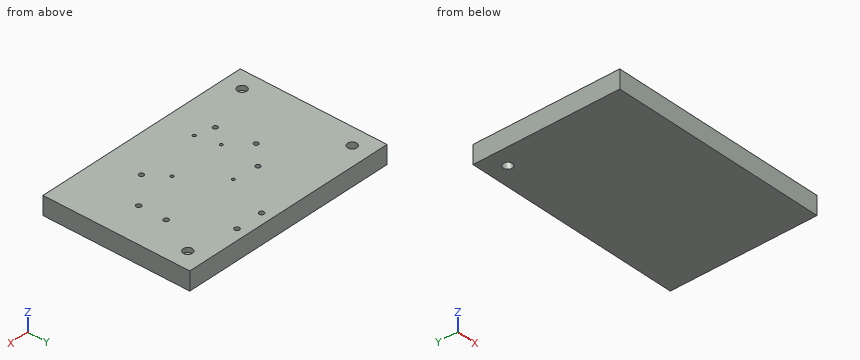
```python
from build123d import *

# Parameters (mm, degrees)
F0_W      = 304.8
F0_H      = 203.2
F1_DEPTH  = 25.4
F2_R      = 6.35
F3_DEPTH  = 6.35
F4_R      = 3.175
F5_DEPTH  = 19.05
F6_R      = 2.0701
F7_DEPTH  = 13.0302
F8_R      = 3.429
F9_DEPTH  = 12.7
F10_R     = 3.175
F11_DEPTH = 6.35
F12_R     = 3.429
F13_DEPTH = 12.7
F14_R     = 2.159
F15_DEPTH = 12.7
F16_R     = 6.35
F17_DEPTH = 25.4


with BuildPart() as f1:
    # F0 (on Top) → F1 (new body)
    with BuildSketch(Plane.XY):
        Rectangle(F0_W, F0_H)
    extrude(amount=F1_DEPTH)

    # F2 (on face) → F3 (cut)
    with BuildSketch(Plane.XY.offset(25.4)):
        with Locations((-127, -76.2)):
            Circle(F2_R)
        with Locations((127, 76.2)):
            Circle(F2_R)
    extrude(amount=-F3_DEPTH, mode=Mode.SUBTRACT)

    # F4 (on face) → F5 (cut)
    with BuildSketch(Plane.XY.offset(25.4)):
        with Locations((-57.15, -50.8)):
            Circle(F4_R)
        with Locations((57.15, -50.8)):
            Circle(F4_R)
        with Locations((-63.5, 0)):
            Circle(F4_R)
    extrude(amount=-F5_DEPTH, mode=Mode.SUBTRACT)

    # F6 (on face) → F7 (cut)
    with BuildSketch(Plane.XY.offset(25.4)):
        with Locations((0, 25.4)):
            Circle(F6_R)
        with Locations((-38.1, -25.4)):
            Circle(F6_R)
        with Locations((38.1, -25.4)):
            Circle(F6_R)
    extrude(amount=-F7_DEPTH, mode=Mode.SUBTRACT)

    # F8 (on face) → F9 (cut)
    with BuildSketch(Plane.XY.offset(25.4)):
        with Locations((25.4, 87.3252)):
            Circle(F8_R)
        with Locations((63.5, 87.3252)):
            Circle(F8_R)
    extrude(amount=-F9_DEPTH, mode=Mode.SUBTRACT)

    # F10 (on face) → F11 (cut)
    with BuildSketch(Plane.XY.offset(25.4)):
        with Locations((-34.6202, 28.575)):
            Circle(F10_R)
    extrude(amount=-F11_DEPTH, mode=Mode.SUBTRACT)

    # F12 (on face) → F13 (cut)
    with BuildSketch(Plane.XY.offset(25.4)):
        with Locations((100.33, 22.225)):
            Circle(F12_R)
        with Locations((100.33, -15.875)):
            Circle(F12_R)
    extrude(amount=-F13_DEPTH, mode=Mode.SUBTRACT)

    # F14 (on face) → F15 (cut)
    with BuildSketch(Plane.XY.offset(25.4)):
        with Locations((-31.75, -57.15)):
            Circle(F14_R)
    extrude(amount=-F15_DEPTH, mode=Mode.SUBTRACT)

    # F16 (on face) → F17 (cut)
    with BuildSketch(Plane.XY.offset(25.4)):
        with Locations((-127, 76.2)):
            Circle(F16_R)
    extrude(amount=-F17_DEPTH, mode=Mode.SUBTRACT)


solid = f1.part
```
The listing builds one solid part. Answer for the finished solid, in the listing's coordinates (mm). Coordinates: 2 decimals unless noted, no trailing zeros. Write each loop counter-clockwise with the first axis right and the second up, starting at its lowest first coordinate (ties: lowest second). Pieces come first, ordered by that corner, then holes. Notation, with made-up numbers: M 48,62 L 85,62 A29 ccw 85,92 Z; hole C -26.75,33 d9. An arc over 180 degrees is marked long. Use a Markdown table: item, result. Add a question column.
1. Section C-C (x = -126.5) is taken. Give the vertices of the cut face in (y, z).
2. Straight lines are drawn through the part: line 1 along Y through (x, z) = (-127, 24.25); line 2 along Y through (x, z) = (-63.5, 18) (3 decimals); line 3 along Y through (x, z) = (127, 20.75). For each, find the intervals that lie inside material, in ascending order. Write a range as [from, to].
3. Section A-A (y = 0) is taken. Give the vertices of the cut face in (x, z) (3 decimals).
4. Section B-B (x = 63.5) is taken. Give the vertices of the cut face in (y, z), plus the area to 3 significant figures.
5. Given P1, Ø7.5, axis at x = -57.15, y = -50.8, coming from the +Z side; P2, Ø2.5, axis at x = -38.1, y = -25.4, coming from the +Z side; P3, Ø1.9, axis at x = -33, y = 30, coming from the +Z side, each flat-ended and moving along its own axis, determine where each tip first touches the part or whether it passes through.
Data:
| question | item | result |
|---|---|---|
| 1 | outline | M -101.6,0 L 69.87,0 L 69.87,25.4 L -69.87,25.4 L -69.87,19.05 L -82.53,19.05 L -82.53,25.4 L -101.6,25.4 Z; M 82.53,0 L 101.6,0 L 101.6,25.4 L 82.53,25.4 Z |
| 2 | line 1 | y = [-101.6, -82.55], [-69.85, 69.85], [82.55, 101.6] |
| 2 | line 2 | y = [-101.6, -3.175], [3.175, 101.6] |
| 2 | line 3 | y = [-101.6, 69.85], [82.55, 101.6] |
| 3 | outline | M -152.4,0 L 152.4,0 L 152.4,25.4 L -60.325,25.4 L -60.325,6.35 L -66.675,6.35 L -66.675,25.4 L -152.4,25.4 Z |
| 4 | outline | M -101.6,0 L 101.6,0 L 101.6,25.4 L 90.75,25.4 L 90.75,12.7 L 83.9,12.7 L 83.9,25.4 L -101.6,25.4 Z |
| 4 | area | 5,070 mm2 |
| 5 | P1 | stops at z = 25.4 |
| 5 | P2 | stops at z = 12.37 |
| 5 | P3 | stops at z = 19.05 |
